Source: CAD feature listing. Evaluate the final solid. Frame: model axes, mm. Face numbers are marked on the shaded views. A direction names the side the tool comes from. Give positions to 0.01 mm unless a question says otherwise; leave off trailing zeros. Loops run counter-clockwise (first coordinate to the right, second up) from the corner with the lowest first, then second, coordinate; pieces in that order, holes last.
```python
from build123d import *

# Parameters (mm, degrees)
F1_DEPTH = 12.7
F2_R     = 2.2733
F3_DEPTH = 3.81
F4_R     = 1.016
F5_DEPTH = 10.616909


with BuildPart() as f1:
    # F0 (on Right) → F1 (new body, symmetric)
    with BuildSketch(Plane.YZ):
        Polygon((6.805909, -12.7), (0, 12.7), (0, -12.7), align=None)
    extrude(amount=F1_DEPTH, both=True)

    # F2 (on face) → F3 (join)
    with BuildSketch(Plane.XZ):
        with Locations((-10.28534, -10.315215)):
            Circle(F2_R)
        with Locations((10.413997, -10.315215)):
            Circle(F2_R)
        with Locations((-10.28534, 2.384785)):
            Circle(F2_R)
        with Locations((10.413997, 2.384785)):
            Circle(F2_R)
    extrude(amount=F3_DEPTH)

    # F4 (on face) → F5 (cut, through all)
    with BuildSketch(Plane.XZ.offset(3.81)):
        with Locations((-10.28534, 2.384785)):
            Circle(F4_R)
        with Locations((-10.28534, -10.345133)):
            Circle(F4_R)
        with Locations((10.44106, 2.384785)):
            Circle(F4_R)
        with Locations((10.44106, -10.345133)):
            Circle(F4_R)
    extrude(amount=-F5_DEPTH, mode=Mode.SUBTRACT)


solid = f1.part
```
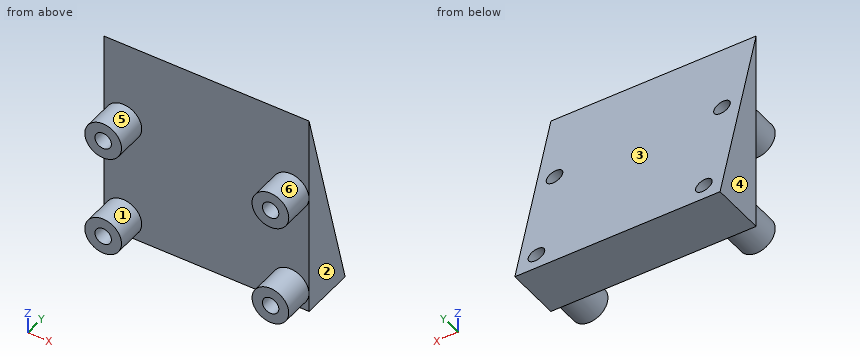
(1) Ray query, line 1 along X through (y, z) = (3.75, -10); line 2 along X through (y, z) = (-2.75, 2.75); line 3 along X through (y, z) = (-3, -10.5). Return the intervals inside material, ascending.
A:
line 1: x = -12.7 to -11.24, -9.33 to 9.49, 11.4 to 12.7
line 2: x = -12.53 to -11.23, -9.34 to -8.04, 8.17 to 9.49, 11.39 to 12.66
line 3: x = -12.55 to -11.29, -9.28 to -8.02, 8.15 to 9.44, 11.45 to 12.68
(2) Reachability of the marked faces 1 and 2 from +Z, -Z, +X, -X, +Y, -Y: full face, straight path, thin tool, end or side. Return the list, or none.
A:
face 1: -Y
face 2: +Z, -Z, +X, +Y, -Y
(3) Section B-B, the plane y = 2.25. Return the cut outline in (x, z).
A:
outline: (-12.7, -12.7) - (12.7, -12.7) - (12.7, 4.3) - (-12.7, 4.3) - close; hole circle Ø2.03 at (-10.29, -10.35); hole circle Ø2.03 at (-10.29, 2.38); hole circle Ø2.03 at (10.44, -10.35); hole circle Ø2.03 at (10.44, 2.38)
(4) Section A-A, the plane z = -10.75. Return the cut outline in (x, y), then the cut area to 3 significant figures.
A:
outline: (-12.7, 0) - (-12.52, 0) - (-12.52, -3.81) - (-11.22, -3.81) - (-11.22, 6.28) - (-12.7, 6.28) - close; (-9.35, -3.81) - (-8.05, -3.81) - (-8.05, 0) - (8.18, 0) - (8.18, -3.81) - (9.51, -3.81) - (9.51, 6.28) - (-9.35, 6.28) - close; (11.37, -3.81) - (12.65, -3.81) - (12.65, 0) - (12.7, 0) - (12.7, 6.28) - (11.37, 6.28) - close
area: 156 mm2
(5) Section C-C, the plane x = 8.5. Return the cut outline in (y, z), then the cut area to 3 significant figures.
A:
outline: (-3.81, -11.54) - (0, -11.54) - (0, -12.7) - (6.81, -12.7) - (0, 12.7) - (0, 3.61) - (-3.81, 3.61) - (-3.81, 1.16) - (0, 1.16) - (0, -9.09) - (-3.81, -9.09) - close
area: 105 mm2
(6) Section D-D, the plane z = 1.75. Return the cut outline in (x, y), then the cut area to 3 significant figures.
A:
outline: (-12.7, 0) - (-12.47, 0) - (-12.47, -3.81) - (-11.08, -3.81) - (-11.08, 2.93) - (-12.7, 2.93) - close; (-9.49, -3.81) - (-8.1, -3.81) - (-8.1, 0) - (8.23, 0) - (8.23, -3.81) - (9.65, -3.81) - (9.65, 2.93) - (-9.49, 2.93) - close; (11.23, -3.81) - (12.6, -3.81) - (12.6, 0) - (12.7, 0) - (12.7, 2.93) - (11.23, 2.93) - close
area: 86.4 mm2
(7) Mould query, pull axis X, two halves, no side actions, for the marked faces 3, 4, 5 and 6. Classes: pulls with the +X half, pulls with the -X half, needs draft (parallel to the pull), parting line crosses it, or undercut.
A:
face 3: needs draft
face 4: pulls with the -X half
face 5: undercut
face 6: undercut
(8) First-contact query: pin 1 (2 mm diameter, centred on x = 4.5, z = 2.5, fed in from -Y); pin 2 (3.5 mm diameter, centred on x = -10.29, z = -10.35, fed in from +Y); pin 3 (3.5 mm diameter, centred on x = -10.29, z = 2.38, fed in from +Y). Flat tips, straight axial feed; report the tip coordinate or a pass-through.
A:
pin 1: stops at y = 0
pin 2: stops at y = 6.65
pin 3: stops at y = 3.23
